Verification items for the finished model (mm, model axes). A direction names the side the tool comes from. Give positions to 0.01 mm unless a question says otherwise; leave off trailing zeros. Loops run counter-clockwise (first coordinate to the right, second up) from the corner with the lowest first, then second, coordinate; pieces in that order, holes last. Notation, with made-up numbers: (-31.5, 28) - (13.5, 28) arc R24 ccw to (13.5, 48) - close; hole circle Ø11 at (29.5, -23.5). An arc over 180 degrees is marked (long way). Use one line per item in the form item = value.
Autodesk Inventor part; units mm, degrees
ref_plane "XY Plane" through (0, 0, 0) normal (0, 0, 1) x (1, 0, 0)
sketch "Sketch1" plane through (0, 0, 0) normal (0, 0, 1) x (1, 0, 0)
  line L0 (0, 137.3747) -> (0, -23.9646)
  line L1 (-192.1248, 0) -> (256.1664, 0)
  arc A0 (-45.1628, 6.4251) -> (-37.5, -10) centre (-37.5, 0) ccw
  arc A1 (37.5, -10) -> (45.1628, 6.4251) centre (37.5, 0) ccw
  arc A2 (12.3157, 77.1386) -> (-12.3157, 77.1386) centre (0, 75) ccw
  arc A3 (-45.1628, 6.4251) -> (-12.3157, 77.1386) centre (-160.104, 102.802) ccw
  arc A4 (12.3157, 77.1386) -> (45.1628, 6.4251) centre (160.104, 102.802) ccw
  line L2 (-37.5, -10) -> (37.5, -10)
  dimension "d0" = 20
  dimension "d1" = 25
  dimension "d2" = 75
  dimension "d3" = 75
  dimension "d4" = 150
extrude "Extrusion1" add sketch "Sketch1" along normal blind 12
sketch "Sketch2" plane through (0, 0, 12) normal (0, 0, 1) x (1, 0, 0)
  arc A0 (-45.1628, 6.4251) -> (-12.3157, 77.1386) centre (-160.104, 102.802) ccw
  arc A1 (-45.1628, 6.4251) -> (-37.5, -10) centre (-37.5, 0) ccw
  line L0 (37.5, -10) -> (-37.5, -10)
  arc A2 (37.5, -10) -> (45.1628, 6.4251) centre (37.5, 0) ccw
  arc A3 (12.3157, 77.1386) -> (45.1628, 6.4251) centre (160.104, 102.802) ccw
  arc A4 (12.3157, 77.1386) -> (-12.3157, 77.1386) centre (0, 75) ccw
  arc A5 (-41.3314, 3.2126) -> (-7.3894, 76.2832) centre (-160.104, 102.802) ccw
  arc A6 (-41.3314, 3.2126) -> (-37.5, -5) centre (-37.5, 0) ccw
  line L1 (-37.5, -5) -> (37.5, -5)
  arc A7 (37.5, -5) -> (41.3314, 3.2126) centre (37.5, 0) ccw
  arc A8 (7.3894, 76.2832) -> (41.3314, 3.2126) centre (160.104, 102.802) ccw
  arc A9 (7.3894, 76.2832) -> (-7.3894, 76.2832) centre (0, 75) ccw
  dimension "d7" = 5
extrude "Extrusion2" add sketch "Sketch2" along normal blind 12 contours A5 A9 A8 A7 L1 A6
sketch "Sketch3" plane through (0, 0, 24) normal (0, 0, 1) x (1, 0, 0)
  arc A0 (5.4189, 75.941) -> (-5.4189, 75.941) centre (0, 75) ccw
  arc A1 (5.4189, 75.941) -> (39.7988, 1.9275) centre (160.104, 102.802) ccw
  arc A2 (37.5, -3) -> (39.7988, 1.9275) centre (37.5, 0) ccw
  line L0 (37.5, -3) -> (-37.5, -3)
  arc A3 (-39.7988, 1.9275) -> (-37.5, -3) centre (-37.5, 0) ccw
  arc A4 (-39.7988, 1.9275) -> (-5.4189, 75.941) centre (-160.104, 102.802) ccw
  line L1 (0, 116.75) -> (0, -19.75)
  line L2 (-57, 0) -> (76, 0)
  dimension "d13" = 3
extrude "Extrusion3" cut sketch "Sketch3" against normal through all
properties part number "redefine"
1. Tool access check on faces 1 (the flat face through (21, 35, 12)), 2 (the cylindrical face through (19.77, 36.99, 17.92)), 3 (the cylindrical face through (0.1, 80.5, 12.2)). Record the directions out of +Z, -Z, +X, -X, +Y, -Y that give a thin tool (end or side, any length) a straight path to the whole face; none if there is none.
Result set:
face_1 = +Z
face_2 = +Z, +X, +Y
face_3 = +Z, -Z
2. Depth check by flat-ended pin: pin 1 Ø2 at (x, z) = (-36.5, 17) entering from +Y; pin 2 Ø3.5 at (x, z) = (4.5, 17.5) entering from -Y; pin 3 Ø7 at (x, z) = (9.5, 10) entering from +Y; pin 4 Ø10 at (x, y) = (-35.5, 37.5) entering from +Z. Enter the tip coordinate at first touch or a pass-through.
Result set:
pin_1 = 10.61
pin_2 = -5
pin_3 = 85.97
pin_4 = through
3. Scan lines: probe 1 along X at (y, z) = (0, 1.5); probe 2 along Y at (x, z) = (20.5, 18); probe 3 along X at (y, z) = (44, 21). Record each from-to range of solid material in increasing order.
Result set:
probe_1 = -47.5 to -40.5, 40.5 to 47.5
probe_2 = -5 to -3, 30.97 to 35.45
probe_3 = -16.69 to -14.53, 14.53 to 16.69
4. Draft check along Y on faces 4 (the cylindrical face through (-23.833, 40.111, 5.916)), 5 (the cylindrical face through (-41.997, -2.186, 17.916)), 6 (the flat face through (1, -3, 12)). Enter one of: released by +Y, released by -Y, zero draft, split by the parting line, or undercut.
Result set:
face_4 = released by +Y
face_5 = split by the parting line
face_6 = undercut
5. Section check C-C, the plane y = 67.5. Record the cut outline in (x, z), then the cut area to 3 significant figures.
Result set:
outline = (-14.32, 0) - (-7.12, 0) - (-7.12, 24) - (-9.18, 24) - (-9.18, 12) - (-14.32, 12) - close; (7.12, 0) - (14.32, 0) - (14.32, 12) - (9.18, 12) - (9.18, 24) - (7.12, 24) - close
area = 222 mm²
6. Section check D-D, the plane z = 16.75. Record the cut outline in (x, y), then the cut area to 3 significant figures.
Result set:
outline = (-41.33, 3.21) arc R5 ccw to (-37.5, -5) - (37.5, -5) arc R5 ccw to (41.33, 3.21) arc R155 cw to (7.39, 76.28) arc R7.5 ccw to (-7.39, 76.28) arc R155 cw to start; hole (-39.8, 1.93) arc R3 ccw to (-37.5, -3) - (37.5, -3) arc R3 ccw to (39.8, 1.93) arc R157 cw to (5.42, 75.94) arc R5.5 ccw to (-5.42, 75.94) arc R157 cw to start
area = 551 mm²
7. Section check B-B, the plane x = 13.5. Record the cut outline in (y, z), then the cut area to 3 significant figures.
Result set:
outline = (-10, 0) - (-3, 0) - (-3, 24) - (-5, 24) - (-5, 12) - (-10, 12) - close; (46.62, 0) - (71.06, 0) - (71.06, 12) - (52.48, 12) - (52.48, 24) - (46.62, 24) - close
area = 472 mm²
8. Section check A-A, the plane z = 2.5. Record the cut outline in (x, y), then the cut area to 3 significant figures.
Result set:
outline = (-45.16, 6.43) arc R10 ccw to (-37.5, -10) - (37.5, -10) arc R10 ccw to (45.16, 6.43) arc R150 cw to (12.32, 77.14) arc R12.5 ccw to (-12.32, 77.14) arc R150 cw to start; hole (-39.8, 1.93) arc R3 ccw to (-37.5, -3) - (37.5, -3) arc R3 ccw to (39.8, 1.93) arc R157 cw to (5.42, 75.94) arc R5.5 ccw to (-5.42, 75.94) arc R157 cw to start
area = 2,040 mm²
